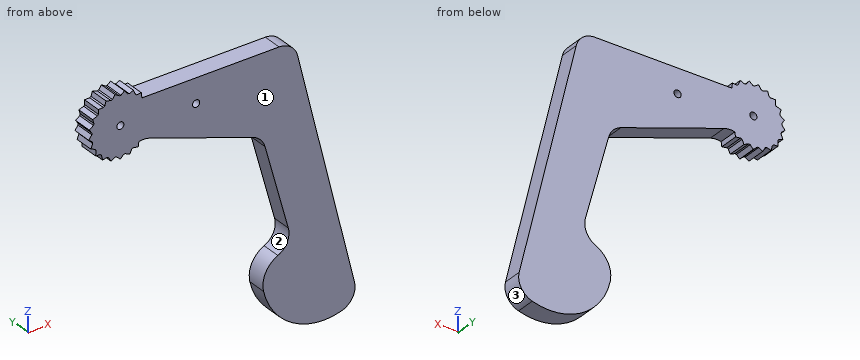
```python
from build123d import *

# Parameters (mm, degrees)
SKETCH1_R           = 1.190625
BOSS_EXTRUDE1_DEPTH = 6.35
FILLET1_R           = 6.35


with BuildPart() as part:
    # Sketch1 → Boss-Extrude1 (new body)
    with BuildSketch(Plane(origin=(0, 0, 0), x_dir=(1, 0, 0), z_dir=(0, 1, 0))):
        with BuildLine():
            Line((-29.821169202, -13.660880054), (20.978830798, -13.660880054))
            Line((20.978830798, -13.660880054), (42.395952597, 74.352713283))
            ThreePointArc((42.395952597, 74.352713283), (23.25712174, 76.338412105), (10.802994012, 61.671014622))
            ThreePointArc((10.802994012, 61.671014622), (13.079862123, 53.776279051), (20.951622371, 51.421206075))
            Line((20.951622371, 51.421206075), (10.410154917, 12.910611329))
            Line((10.410154917, 12.910611329), (-29.996286473, -0.999994782))
            ThreePointArc((-29.996286473, -0.999994782), (-30.398101975, -0.586570963), (-30.824193291, -0.198213985))
            Line((-30.824193291, -0.198213985), (-31.044454647, 1.322241923))
            Line((-31.044454647, 1.322241923), (-32.73765618, 1.076955714))
            ThreePointArc((-32.73765618, 1.076955714), (-32.976313311, 1.193094592), (-33.218113701, 1.302538808))
            Line((-33.218113701, 1.302538808), (-33.874715297, 2.691486458))
            Line((-33.874715297, 2.691486458), (-35.421467347, 1.960285492))
            ThreePointArc((-35.421467347, 1.960285492), (-35.683694268, 2.001303864), (-35.946962256, 2.035000026))
            Line((-35.946962256, 2.035000026), (-36.982128516, 3.170223372))
            Line((-36.982128516, 3.170223372), (-38.246329537, 2.017447359))
            ThreePointArc((-38.246329537, 2.017447359), (-38.509052422, 1.979735943), (-38.770622576, 1.934719064))
            Line((-38.770622576, 1.934719064), (-40.093267325, 2.716327725))
            Line((-40.093267325, 2.716327725), (-40.963677954, 1.243411538))
            ThreePointArc((-40.963677954, 1.243411538), (-41.203779335, 1.130288631), (-41.440635618, 1.010519829))
            Line((-41.440635618, 1.010519829), (-42.934376923, 1.369738627))
            Line((-42.934376923, 1.369738627), (-43.334408136, -0.293713141))
            ThreePointArc((-43.334408136, -0.293713141), (-43.530761052, -0.472293647), (-43.722062046, -0.656275697))
            Line((-43.722062046, -0.656275697), (-45.255462875, -0.751055081))
            Line((-45.255462875, -0.751055081), (-45.149915191, -2.458672264))
            ThreePointArc((-45.149915191, -2.458672264), (-45.285242191, -2.686996744), (-45.414154972, -2.919003123))
            Line((-45.414154972, -2.919003123), (-46.852288576, -3.459440878))
            Line((-46.852288576, -3.459440878), (-46.250449331, -5.060967113))
            ThreePointArc((-46.250449331, -5.060967113), (-46.312842744, -5.318944878), (-46.368024039, -5.57856092))
            Line((-46.368024039, -5.57856092), (-47.58434641, -6.517102938))
            Line((-47.58434641, -6.517102938), (-46.539172541, -7.871616999))
            ThreePointArc((-46.539172541, -7.871616999), (-46.523142255, -8.136548112), (-46.499736562, -8.400929727))
            Line((-46.499736562, -8.400929727), (-47.387221268, -9.654991978))
            Line((-47.387221268, -9.654991978), (-45.990679537, -10.643307692))
            ThreePointArc((-45.990679537, -10.643307692), (-45.897636087, -10.89188038), (-45.797702915, -11.137764145))
            Line((-45.797702915, -11.137764145), (-46.278258552, -12.596999395))
            Line((-46.278258552, -12.596999395), (-44.653233223, -13.132153052))
            ThreePointArc((-44.653233223, -13.132153052), (-44.491363673, -13.34249495), (-44.323696325, -13.548245102))
            Line((-44.323696325, -13.548245102), (-44.355037921, -15.084252569))
            Line((-44.355037921, -15.084252569), (-42.644517948, -15.11915502))
            ThreePointArc((-42.644517948, -15.11915502), (-42.428065496, -15.272757758), (-42.207417329, -15.420269965))
            Line((-42.207417329, -15.420269965), (-41.78678708, -16.897893539))
            Line((-41.78678708, -16.897893539), (-40.141284249, -16.429473653))
            ThreePointArc((-40.141284249, -16.429473653), (-39.889294943, -16.512821445), (-39.635081193, -16.589115838))
            Line((-39.635081193, -16.589115838), (-38.799491125, -17.878336715))
            Line((-38.799491125, -17.878336715), (-37.363796242, -16.947811616))
            ThreePointArc((-37.363796242, -16.947811616), (-37.098443082, -16.953570537), (-36.833032482, -16.951933832))
            Line((-36.833032482, -16.951933832), (-35.656007696, -17.939311107))
            Line((-35.656007696, -17.939311107), (-34.556450183, -16.628559402))
            ThreePointArc((-34.556450183, -16.628559402), (-34.301082079, -16.556222714), (-34.047828595, -16.476798928))
            Line((-34.047828595, -16.476798928), (-32.632937655, -17.075451466))
            Line((-32.632937655, -17.075451466), (-31.966269592, -15.499808597))
            ThreePointArc((-31.966269592, -15.499808597), (-31.743356851, -15.355741339), (-31.52454472, -15.205519116))
            Line((-31.52454472, -15.205519116), (-29.996286473, -15.362770384))
            Line((-29.996286473, -15.362770384), (-29.821169202, -13.660880054))
        make_face()
        with Locations(Location((-37.024468694, -7.428857796, 0), (0, 0, 270))):
            Circle(SKETCH1_R, mode=Mode.SUBTRACT)
        with Locations(Location((-11.697065196, -5.509839295, 0), (0, 0, 270))):
            Circle(SKETCH1_R, mode=Mode.SUBTRACT)
    extrude(amount=BOSS_EXTRUDE1_DEPTH)

    # Fillet1
    # the kernel refuses this fillet: 6.35 mm, written as the material it adds along each edge
    with BuildSketch(Plane(origin=(-29.996286473, 0, 0.999994782), x_dir=(0.9455362039998026, 0, -0.3255169533613324), z_dir=(0, 1, 0))) as fillet1_piece_1:
        with BuildLine():
            CenterArc((2.941509547, 6.35), FILLET1_R, 236.94754351, 33.05245649)
            ThreePointArc((-0.521822628, 1.027610476), (-0.245354643, 0.521704946), (0, 0))
            Line((0, 0), (2.941509547, 0))
        make_face()
    extrude(amount=6.35)
    with BuildSketch(Plane(origin=(10.410154917, 0, -12.910611329), x_dir=(0.2640166060846216, 0, -0.9645181344648517), z_dir=(0, 1, 0))) as fillet1_piece_2:
        with BuildLine():
            CenterArc((FILLET1_R * 0.528295396262, FILLET1_R), FILLET1_R, 214.305424952, 55.694575048)
            Line((-FILLET1_R * 0.297749538039, FILLET1_R * 0.436395735897), (0, 0))
            Line((0, 0), (FILLET1_R * 0.528295396262, 0))
        make_face()
    extrude(amount=6.35)
    with BuildSketch(Plane(origin=(20.951622371, 0, -51.421206075), x_dir=(-0.9938958560926382, 0, -0.11032237869934564), z_dir=(0, 1, 0))) as fillet1_piece_3:
        with BuildLine():
            CenterArc((7.380811015, 6.028648653), FILLET1_R, 171.02537205, 80.668791662)
            Line((1.108550782, 7.019230085), (0, 0))
            ThreePointArc((0, 0), (2.693172408, 0.433927926), (5.386344816, 0))
        make_face()
    extrude(amount=6.35)
    # the kernel refuses this fillet: 6.35 mm, written as the material it takes off along each edge
    with BuildSketch(Plane(origin=(20.978830798, -12.475246836, 13.660880054), x_dir=(-1, 0, 0), z_dir=(0, 1, 0))) as fillet1_2_piece_1:
        with BuildLine():
            CenterArc((FILLET1_R * 0.785842320361, -FILLET1_R), FILLET1_R, 90, 76.323524065)
            Line((-FILLET1_R * 0.185803956952, -FILLET1_R * 0.763560765133), (0, 0))
            Line((0, 0), (FILLET1_R * 0.785842320361, 0))
        make_face()
    extrude(amount=31.300493671, mode=Mode.SUBTRACT)
    with BuildSketch(Plane(origin=(42.395952597, -15.381047636, -74.352713283), x_dir=(-0.23643923486666696, 0, 0.9716462773127189), z_dir=(0, 1, 0))) as fillet1_2_piece_2:
        with BuildLine():
            CenterArc((5.118829866, -6.35), FILLET1_R, 90, 87.108005414)
            ThreePointArc((-1.223082878, -6.029620925), (-0.837554928, -2.968964591), (0, 0))
            Line((0, 0), (5.118829866, 0))
        make_face()
    extrude(amount=37.112095273, mode=Mode.SUBTRACT)


solid = part.part
```
For this review, take the finished solid that the model builds, in its own axes (mm). Face numbers are marked on the shaded views. Round coordinates to 2 decimals unless told otherwise and drop trailing zeros. Order: outer loops, then holes, each group sorted by start corner. A loop starts at its lowest first (then second) coordinate and runs counter-clockwise, first axis right, second up. Notation, with made-up numbers: (-8, 45.5) -> (43, 45.5) arc R15 cw to (43, 65.5) -> close; hole circle Ø11 at (77, 60). An arc over 180 degrees is marked (long way). Use a Markdown table: item, result.
Item 1: For line 1 along Z through (x, y) = (-42.5, 0.5); line 2 along X through (y, z) = (3.25, -71); line 3 along Z through (x, y) = (-27.5, 1.5), list the stretches that pass through material, from the lowest coordinate up. Write a range as [from, to].
Resolved:
| item | result |
|---|---|
| line 1 | z = [-1.27, 15.22] |
| line 2 | x = [15.61, 41.36] |
| line 3 | z = [0.13, 13.66] |
Item 2: For pin 1 (2 mm diameter, centred on x = 19, y = 5, fed in from -Z); pin 2 (3 mm diameter, centred on x = -3.5, y = 3.5, fed in from +Z); pin 3 (3 mm diameter, centred on y = 1.5, z = -57.5, fed in from +X), all flat-tipped, find the tip position at first contact; note any pin that passes through.
Resolved:
| item | result |
|---|---|
| pin 1 | stops at z = -74.68 |
| pin 2 | stops at z = 13.66 |
| pin 3 | stops at x = 38.66 |
Item 3: Take a section at A-A (x = -7). State the section outline as (y, z) points, plus the area to 3 significant figures.
Resolved:
| item | result |
|---|---|
| outline | (0, -6.92) -> (6.35, -6.92) -> (6.35, 13.66) -> (0, 13.66) -> close |
| area | 131 mm² |
Item 4: Take a section at B-B (y = 2). State how many separate pieces and enclosed holes the cut face has, plus the area to 3 significant figures.
Resolved:
| item | result |
|---|---|
| separate pieces | 1 |
| enclosed holes | 2 |
| area | 2,730 mm² |
Item 5: Draft analysis for pull direction Z (two halves, no side actions). For the marked faces 1, 2 and 3, state which applies: +Z half, -Z half, draft (parallel to the pull), parting line (faces both ways), or undercut.
Resolved:
| item | result |
|---|---|
| face 1 | draft |
| face 2 | undercut |
| face 3 | parting line |
Item 6: Take a section at C-C (z = -42). State the section outline as (x, y) points, plus the area to 3 significant figures.
Resolved:
| item | result |
|---|---|
| outline | (18.37, 0) -> (34.52, 0) -> (34.52, 6.35) -> (18.37, 6.35) -> close |
| area | 103 mm² |
